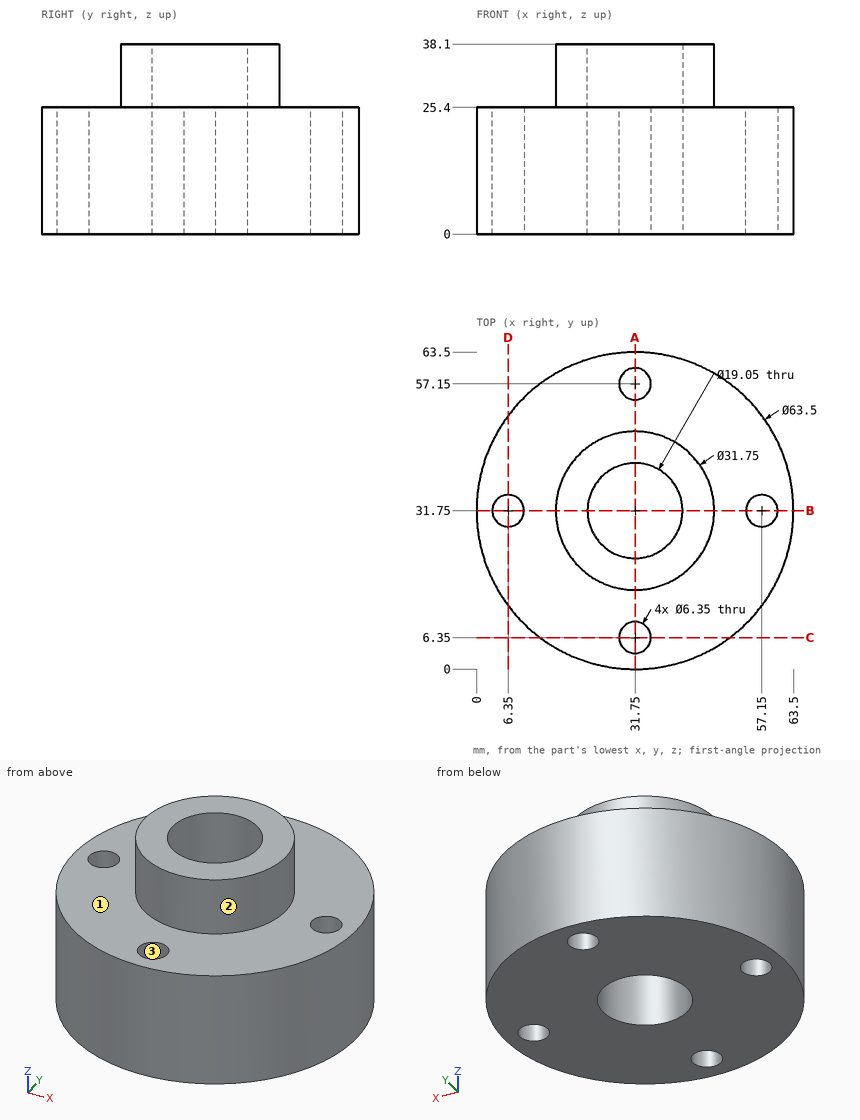
Design review of the part shown in the three views and the two pictorial views. Dimensions are in mm from the part's minimum x, y and z. Round coordinates to 2 decimals unless told otherwise and drop trailing zeros. Write each loop counter-clockwise with the first axis right and the second up, starting at its lowest first coordinate (ties: lowest second). Pieces come first, ordered by that corner, then holes.
Item 1: For pin 1 Ø12 at (x, z) = (41.5, 10) entering from -Y; pin 2 Ø5 at (x, y) = (6.35, 31.75) entering from +Z; pin 3 Ø1.5 at (x, z) = (21.5, 23.5) entering from +Y; pin 4 Ø8 at (x, z) = (17.5, 32.5) entering from -Y, all flat-tipped, find the tip position at first contact; note any pin that passes through.
Item 2: Wall thickness on L1, parallel to Y at x = 31.75, z = 8 (3 decimals); L2, parallel to X at y = 31, z = 7; L3, parallel to X at y = 29, z = 23: over which ranges is each line inside the solid? List them lowest first.
Item 3: Consider section A-A on x = 31.75. Give the boundary of the cut face in (y, z) (3 decimals), and give its area (3 significant figures).
Item 4: Consider section C-C on y = 6.35. Give the boundary of the cut face in (x, z) (3 decimals).
Item 5: Draft analysis for pull direction X (two halves, no side actions). For the marked faces 1, 2 and 3, state which applies: released by +X, released by -X, zero draft, split by the parting line, or undercut.
Check values:
1. pin 1: stops at y = 0.22
1. pin 2: passes through
1. pin 3: stops at y = 62.05
1. pin 4: stops at y = 19.63
2. L1: y = 0 to 3.175, 9.525 to 22.225, 41.275 to 53.975, 60.325 to 63.5
2. L2: x = 0.01 to 3.26, 9.44 to 22.25, 41.25 to 54.06, 60.24 to 63.49
2. L3: x = 0.12 to 4.76, 7.94 to 22.63, 40.87 to 55.56, 58.74 to 63.38
3. outline: (0, 0) - (3.175, 0) - (3.175, 25.4) - (0, 25.4) - close; (9.525, 0) - (22.225, 0) - (22.225, 38.1) - (15.875, 38.1) - (15.875, 25.4) - (9.525, 25.4) - close; (41.275, 0) - (53.975, 0) - (53.975, 25.4) - (47.625, 25.4) - (47.625, 38.1) - (41.275, 38.1) - close; (60.325, 0) - (63.5, 0) - (63.5, 25.4) - (60.325, 25.4) - close
3. area: 968 mm2
4. outline: (12.7, 0) - (28.575, 0) - (28.575, 25.4) - (12.7, 25.4) - close; (34.925, 0) - (50.8, 0) - (50.8, 25.4) - (34.925, 25.4) - close
5. face 1: zero draft
5. face 2: split by the parting line
5. face 3: undercut
